Model file for the job. Use its own axes, mm. A direction names the side the tool comes from. Coordinates: 2 decimals unless noted, no trailing zeros. Order: outer loops, then holes, each group sorted by start corner. A loop starts at its lowest first (then second) coordinate and runs counter-clockwise, first axis right, second up. Notation, with made-up numbers: (-19.5, -17.75) -> (3.5, -17.75) arc R15 ccw to (3.5, 5.25) -> close; hole circle Ø8 at (6.25, 89). An arc over 180 degrees is marked (long way). Return JSON: item names as keys, results as strings. Group by question number.
1) Probe line 1 (Z direction, x = -2, y = -12.5); line 2 (X direction, y = -16.5, z = -2); line 3 (Y direction, x = 11, z = 9.5). List the from-to ranges inside material, lowest first.
2) Cut at A-A (y = -13.5). Write the cut outline in (x, z), and give its area (3 significant figures).
3) Cut at B-B (z = 2.5). Write the cut outline in (x, y).
4) Flat gauge pins, fed straight in: pin 1 (5 mm diameter, centred on x = 3.5, z = 16, fed in from +Y); pin 2 (2 mm diameter, centred on y = -5, z = -3.5, fed in from -X); pin 3 (5 mm diameter, centred on y = -20, z = 16.5, fed in from -X). Where does each tip first touch, or does it go through?
5) Which spindle directions (+Z, -Z, +X, -X, +Y, -Y) get a long thin tool onto all of the face, cutting with end or side? Do faces 1 (the flat face through (-31.75, -32, 0)), 2 (the flat face through (0, -10.16, 14)), 3 (the flat face through (0, -18, 8.89)). Say none if no direction does.
6) Pull direction Z, two halves, no side cores. Call faces 4 (the flat face through (12.7, -10, 0)), 5 (the flat face through (7, -23, -19.05)), 6 (the flat face through (0, -10.16, -14)): +Z half, -Z half, draft (parallel to the pull), parting line (faces both ways), or undercut.
7) Cut at C-C (x = -0.5). Write the cut outline in (y, z), and give its area (3 significant figures).
8) Cut at D-D (x = -26). Write the cut outline in (y, z), and give its area (3 significant figures).
from build123d import *

# Parameters (mm, degrees)
F0_W     = 63.5
F0_H     = 38.1
F1_DEPTH = 38.1
F2_W     = 25.4
F2_H     = 10.16
F3_DEPTH = 10.16
F5_DEPTH = 25.4


with BuildPart() as f1:
    # F0 (on Front) → F1 (new body)
    with BuildSketch(Plane.XZ):
        Rectangle(F0_W, F0_H)
    extrude(amount=F1_DEPTH)

    # F2 (on face) → F3 (cut)
    with BuildSketch(Plane(origin=(0, 0, 0), x_dir=(-1, 0, 0), z_dir=(0, 1, 0))):
        with Locations((0, 13.97)):
            Rectangle(F2_W, F2_H)
        with Locations((0, -13.97)):
            Rectangle(F2_W, F2_H)
    extrude(amount=-F3_DEPTH, mode=Mode.SUBTRACT)

    # F4 (on face) → F5 (cut)
    with BuildSketch(Plane(origin=(0, 0, 0), x_dir=(-1, 0, 0), z_dir=(0, 1, 0))):
        Polygon((31.75, -19.05), (31.75, 19.05), (12.7, 19.05), (12.7, 8.89), (-12.7, 8.89), (-12.7, -8.89), (12.7, -8.89), (12.7, -19.05), align=None)
    extrude(amount=-F5_DEPTH, mode=Mode.SUBTRACT)


solid = f1.part
Answers below:
{
 "1": {"line 1": "z = -19.05 to -8.89, 8.89 to 19.05", "line 2": "x = 12.7 to 31.75", "line 3": "y = -38.1 to -10.16"},
 "2": {"outline": "(-12.7, -19.05) -> (31.75, -19.05) -> (31.75, 19.05) -> (-12.7, 19.05) -> (-12.7, 8.89) -> (12.7, 8.89) -> (12.7, -8.89) -> (-12.7, -8.89) -> close", "area": "1,240 mm^2"},
 "3": {"outline": "(-31.75, -38.1) -> (31.75, -38.1) -> (31.75, 0) -> (12.7, 0) -> (12.7, -25.4) -> (-31.75, -25.4) -> close"},
 "4": {"pin 1": "stops at y = -10.16", "pin 2": "stops at x = 12.7", "pin 3": "stops at x = -12.7"},
 "5": {"face 1": "+Z, -Z, -X, +Y, -Y", "face 2": "+Z, -Z, -X, +Y", "face 3": "-X, +Y"},
 "6": {"face 4": "undercut", "face 5": "-Z half", "face 6": "draft"},
 "7": {"outline": "(-38.1, -19.05) -> (-10.16, -19.05) -> (-10.16, -8.89) -> (-25.4, -8.89) -> (-25.4, 8.89) -> (-10.16, 8.89) -> (-10.16, 19.05) -> (-38.1, 19.05) -> close", "area": "794 mm^2"},
 "8": {"outline": "(-38.1, -19.05) -> (-25.4, -19.05) -> (-25.4, 19.05) -> (-38.1, 19.05) -> close", "area": "484 mm^2"}
}
